Read the model definition and answer for the solid it produces. Units are mm, in the model's axes. A direction names the side the tool comes from. Give positions to 0.01 mm unless a question says otherwise; leave off trailing zeros. Order: outer loops, then holes, each group sorted by start corner. A loop starts at its lowest first (then second) coordinate and runs counter-clockwise, first axis right, second up. Notation, with made-up numbers: M 50.5,-30.5 L 93.5,-30.5 A18 ccw 93.5,-26.5 Z; hole C 12,28.5 d7. An arc over 180 degrees is marked long. One line per item, written item: value.
from build123d import *

# Parameters (mm, degrees)
FILLET_1_R               = 3
CUT_EXTRUDE_1_REACH      = 28.958
SKETCH_2_W               = 10.643557705
SKETCH_2_H               = 9.097593034
PATTERN_CIRCULAR_1_COUNT = 4


with BuildPart() as part:
    # ｽｹｯﾁ1 → 回転1 (revolve)
    with BuildSketch(Plane(origin=(0, 0, 0), x_dir=(0, 0, -1), z_dir=(1, 0, 0)), mode=Mode.PRIVATE) as revolve_1_sk:
        Polygon((0, 7.5), (2, 7.5), (5, 8.5), (20, 6), (20, 0), (16.5, 0), (16.5, 5), (6.5, 6.5), (1.5, 5), (-1.5, 5), (-1.5, 11.5), (0, 11.5), align=None)
    revolve(revolve_1_sk.sketch.rotate(Axis((0, 0, 0), (0, 0, 1)), 90), axis=Axis((0, 0, 0), (0, 0, 1)))

    # ﾌｨﾚｯﾄ1
    fillet_1_edges = [part.edges().sort_by_distance(p)[0] for p in [
        (6, 0, -20),
    ]]
    fillet(fillet_1_edges, radius=FILLET_1_R)

    # ｶｯﾄ - 押し出し1: up to this face of the body (flat: up to its plane)
    cut_extrude_1_end = Plane(part.part.faces().sort_by_distance((11.174730881, 0, 0))[0])
    # ｽｹｯﾁ2 → ｶｯﾄ - 押し出し1 (cut, up to the picked face)
    with BuildSketch(Plane(origin=(0, 0, -20), x_dir=(-1, 0, 0), z_dir=(0, 0, -1)), mode=Mode.PRIVATE) as cut_extrude_1_sk1:
        with Locations((8.321778852, 7.548796517)):
            Rectangle(SKETCH_2_W, SKETCH_2_H)
    cut_extrude_1_tool1 = split(extrude(cut_extrude_1_sk1.sketch, amount=-CUT_EXTRUDE_1_REACH, mode=Mode.PRIVATE), bisect_by=cut_extrude_1_end, keep=Keep.BOTH, mode=Mode.PRIVATE)
    cut_extrude_1 = cut_extrude_1_tool1.solids().sort_by(Axis((-8.321779, 7.548797, -20), (0, 0, 1)))[0]
    add(cut_extrude_1, mode=Mode.SUBTRACT)

    # 円形ﾊﾟﾀｰﾝ1: ｶｯﾄ - 押し出し1 ×4 about axis
    pattern_circular_1_axis = Axis((0, 0, 0), (0, 0, 1))
    for i in range(1, PATTERN_CIRCULAR_1_COUNT):
        add(cut_extrude_1.rotate(pattern_circular_1_axis, i * 360 / PATTERN_CIRCULAR_1_COUNT), mode=Mode.SUBTRACT)


solid = part.part
1) Each of these flat-tipped pins is pushed along its axis until it touches: pin 1 Ø4 at (x, z) = (-6.5, -7.5) entering from +Y; pin 2 Ø3 at (x, y) = (0, -0.5) entering from +Z; pin 3 Ø4 at (y, z) = (-6, -11.5) entering from -X; pin 4 Ø8 at (x, z) = (2.5, -1) entering from +Y. Where does it stop, or does it pass through?
Reported:
pin 1: stops at y = 3
pin 2: stops at z = -16.5
pin 3: stops at x = -3
pin 4: stops at y = 11.5
2) Which of the six approach directions +Z, -Z, +X, -X, +Y, -Y give full straight-line access (tool end or side, diameter ignored) to faces 5 (the face through (-5.4, 3, -10.1)), 6 (the face through (0.052, 5.739, -3.965)), 7 (the face through (8, 0, -3.5))?
Reported:
face 5: -Z, -X, +Y
face 6: none
face 7: +X
3) Consider probe 1 along Y at (x, z) = (0, 0.55); probe 2 along Z at (x, y) = (-6.25, -5.25); probe 3 along Y at (x, z) = (2.25, -4). Determine where each line is inside the solid, lowest interval first.
Reported:
probe 1: y = -11.5 to -5, 5 to 11.5
probe 2: z = 0 to 1.5
probe 3: y = -7.85 to -5.29, 5.29 to 7.85
4) Find section D-D, the plane z = -18.25. Write down the section's boundary in (x, y), plus the area to 3 significant figures.
Reported:
outline: M -5.41,-3 L -3,-3 L -3,-5.41 A6.19 ccw 3,-5.41 L 3,-3 L 5.41,-3 A6.19 ccw 5.41,3 L 3,3 L 3,5.41 A6.19 ccw -3,5.41 L -3,3 L -5.41,3 A6.19 ccw Z
area: 106 mm^2
5) Find section B-B, the plane y = 0. Write down the section's boundary in (x, z), plus the area to 3 significant figures.
Reported:
outline: M -11.5,0 L -7.5,0 L -7.5,-2 L -8.5,-5 L -6.42,-17.49 A3 ccw -3.46,-20 L 3.46,-20 A3 ccw 6.42,-17.49 L 8.5,-5 L 7.5,-2 L 7.5,0 L 11.5,0 L 11.5,1.5 L 5,1.5 L 5,-1.5 L 6.5,-6.5 L 5,-16.5 L -5,-16.5 L -6.5,-6.5 L -5,-1.5 L -5,1.5 L -11.5,1.5 Z
area: 125 mm^2
6) Find section A-A, the plane z = -1. Write down the section's boundary in (x, y).
Reported:
outline: M -6.87,-3 L -4,-3 A5 cw -4,3 L -6.87,3 A7.5 ccw Z; M -3,-6.87 A7.5 ccw 3,-6.87 L 3,-4 A5 cw -3,-4 Z; M -3,4 A5 cw 3,4 L 3,6.87 A7.5 ccw -3,6.87 Z; M 4,-3 L 6.87,-3 A7.5 ccw 6.87,3 L 4,3 A5 cw Z
7) Determine the mould class of faces 1 (the face through (3, -5.4, -10.1)), 2 (the face through (5.4, 3, -10.1)), 3 (the face through (0, 8, -3.5)), 4 (the face through (-0.05, -5.76, -11.43)) for opening direction X: +X half, -X half, draft (parallel to the pull), parting line (faces both ways), or undercut.
Reported:
face 1: +X half
face 2: draft
face 3: parting line
face 4: undercut
